from build123d import *

# Parameters (mm, degrees)
SKETCH1_W           = 38
SKETCH1_H           = 24.5
SKETCH1_R           = 8.3
BOSS_EXTRUDE1_DEPTH = 5
FILLET1_R           = 15
FILLET2_R           = 1
CHAMFER1_SIZE       = 0.75
SKETCH3_W           = 1.267094865
SKETCH3_H           = 1.151259449


with BuildPart() as part:
    # Sketch1 → Boss-Extrude1 (new body)
    with BuildSketch(Plane(origin=(0, 0, 0), x_dir=(1, 0, 0), z_dir=(0, 1, 0))):
        Rectangle(SKETCH1_W, SKETCH1_H)
        with Locations(Location((0, 0, 0), (0, 0, 270))):
            Circle(SKETCH1_R, mode=Mode.SUBTRACT)
    extrude(amount=BOSS_EXTRUDE1_DEPTH)

    # Fillet1
    fillet1_edges = [part.edges().sort_by_distance(p)[0] for p in [
        (19, 2.5, 12.25),
        (-19, 2.5, 12.25),
    ]]
    fillet(fillet1_edges, radius=FILLET1_R)

    # Fillet2
    fillet2_edges = [part.edges().sort_by_distance(p)[0] for p in [
        (-19, 2.5, -12.25),
        (19, 2.5, -12.25),
    ]]
    fillet(fillet2_edges, radius=FILLET2_R)

    # Chamfer1
    chamfer1_edges = [part.edges().sort_by_distance(p)[0] for p in [
        (0, 5, -8.3),
    ]]
    chamfer(chamfer1_edges, length=CHAMFER1_SIZE)

    # o-ring: sweep along a path in Sketch4
    with BuildLine(Plane(origin=(0, 5, 0), x_dir=(1, 0, 0), z_dir=(0, 1, 0))) as o_ring_path:
        CenterArc((0, 0), 11, 0, 360)
    # Sketch3 → o-ring (sweep, cut)
    with BuildSketch(Plane.XY):
        with Locations((-11.133547433, 4.975629725)):
            Rectangle(SKETCH3_W, SKETCH3_H)
    sweep(path=o_ring_path.line, mode=Mode.SUBTRACT)


solid = part.part
Can you work these out from the model? Positions are in its coordinate system, mm. A direction names the side the tool comes from. Round coordinates to 2 decimals unless told otherwise and drop trailing zeros. Write each loop counter-clockwise with the first axis right and the second up, starting at its lowest first coordinate (ties: lowest second). Pieces come first, ordered by that corner, then holes. Notation, with made-up numbers: M 55.25,87 L 61.25,87 A10 ccw 61.25,102 Z; hole C 65,57 d9. An arc over 180 degrees is marked long. Use a Markdown table: item, result.
Item 1: For pin 1 Ø8 at (x, z) = (-5.5, 2.5) entering from +Y; pin 2 Ø1 at (y, z) = (4, 4) entering from +X, each with a flat end and sliding along its axis, tell me the tip position at first contact or that it passes through.
Found:
| item | result |
|---|---|
| pin 1 | stops at y = 5 |
| pin 2 | stops at x = 17.64 |
Item 2: I want a section at B-B (x = 15.5). List the corners of the cut face in (y, z) for me.
Found:
| item | result |
|---|---|
| outline | M 0,-12.25 L 5,-12.25 L 5,6.88 L 0,6.88 Z |
Item 3: I want a section at A-A (y = 0.9). List the corners of the cut face in (x, z) for me, and give its area (3 significant figures).
Found:
| item | result |
|---|---|
| outline | M -19,-11.25 A1 ccw -18,-12.25 L 18,-12.25 A1 ccw 19,-11.25 L 19,-2.75 A15 ccw 4,12.25 L -4,12.25 A15 ccw -19,-2.75 Z; hole C 0,0 d16.6 |
| area | 618 mm2 |
Item 4: If I drill on line 1 along Z through (x, y) = (0, 4.7); line 2 along Z through (x, y) = (0, 4.8); line 3 along X through (y, z) = (3.05, -2), over which ranges is the centre line in solid material (lowest first)? Write a range as [from, to].
Found:
| item | result |
|---|---|
| line 1 | z = [-12.25, -11.77], [-10.5, -8.75], [8.75, 10.5], [11.77, 12.25] |
| line 2 | z = [-12.25, -11.77], [-10.5, -8.85], [8.85, 10.5], [11.77, 12.25] |
| line 3 | x = [-18.98, -8.06], [8.06, 18.98] |
Item 5: We'd pull the mould along X, two halves only. Please class faces 1 (the face through (14.49, 2.54, 7.97)), 2 (the face through (0, 2, 12.25)), 3 (the face through (-5.05, 2.095, -6.587)): released by +X, released by -X, zero draft, split by the parting line, or undercut.
Found:
| item | result |
|---|---|
| face 1 | released by +X |
| face 2 | zero draft |
| face 3 | undercut |
Item 6: Which directions (+Z, -Z, +X, -X, +Y, -Y) give clear straight access to the entire face, cutting with the end or side of a thin tool? Please do faces 4 (the face through (-2.28, 4.7, 10.25)), 5 (the face through (-4.5, 5, -11.1)).
Found:
| item | result |
|---|---|
| face 4 | +Y |
| face 5 | +Z, -Z, +X, -X, +Y |
